Autodesk Inventor part; units mm, degrees
ref_plane "YZ Plane" through (0, 0, 0) normal (1, 0, 0) x (0, 1, 0)
ref_plane "XZ Plane" through (0, 0, 0) normal (0, 1, 0) x (-1, 0, 0)
ref_plane "XY Plane" through (0, 0, 0) normal (0, 0, 1) x (1, 0, 0)
sketch "Sketch1" plane through (0, 0, 0) normal (0, 1, 0) x (-1, 0, 0)
  line L0 (-3, -29) -> (3, -29)
  line L1 (3, -29) -> (3, 29)
  line L2 (3, 29) -> (-3, 29)
  line L3 (-3, 29) -> (-3, -29)
  line L4 (-3, -29) -> (3, 29) construction
  line L5 (3, -29) -> (-3, 29) construction
  point P0 (0, 0)
  dimension "d0" = 58
  dimension "d1" = 6
extrude "Main Body Extrusion" add sketch "Sketch1" along normal blind 4
sketch "Sketch2" plane through (0, 4, 0) normal (0, 1, 0) x (1, 0, 0)
  line L0 (-3, 29) -> (-3, -29)
  line L1 (3, -29) -> (3, 29)
  line L2 (-3, -29) -> (3, -29)
  line L3 (3, -29) -> (3, -23)
  line L4 (3, -23) -> (-3, -23)
  line L5 (-3, -23) -> (-3, -29)
  line L6 (3, 29) -> (-3, 29)
  line L7 (-3, 29) -> (3, 29)
  line L8 (3, 29) -> (3, 23)
  line L9 (3, 23) -> (-3, 23)
  line L10 (-3, 23) -> (-3, 29)
  point P0 (0, 0)
  dimension "d4" = 6
  dimension "d5" = 6
  dimension "d6" = 6
  dimension "d7" = 6
  dimension "d8" = 6
extrude "Side Beams Extrusion" add sketch "Sketch2" along normal blind 20 contours L6 L1 L9 L0 | L4 L1 L2 L0
sketch "Sketch3" plane through (0, 24, 0) normal (0, 1, 0) x (1, 0, 0)
  line L0 (-3, 23) -> (-3, -23)
  line L1 (3, -23) -> (3, 23)
  circle A0 centre (0, 26) radius 2
  line L2 (-3, 23) -> (3, 23)
  line L3 (3, 29) -> (-3, 29)
  circle A1 centre (0, -26) radius 2
  line L4 (-3, -29) -> (3, -29)
  line L5 (3, -29) -> (3, -23)
  point P0 (0, 0)
  dimension "d11" = 6
  dimension "d12" = 4
  dimension "d13" = 3
  dimension "d14" = 6
  dimension "d15" = 3
  dimension "d16" = 4
  dimension "d17" = 3
  dimension "d18" = 3
extrude "Extrusion3" cut sketch "Sketch3" against normal blind 7
fillet "Fillet1" radius 2 10 edges at (-3, 14, -23) (-3, 12, -29) (-3, 4, 0) (3, 4, 0) (-3, 12, 29) (-3, 14, 23) (3, 12, 29) (3, 14, -23) (3, 12, -29) (3, 14, 23)
equation "\"d5\" = d4"
equation "\"d6\" = d4"
equation "\"d7\" = d4"
equation "\"d8\" = d4"
equation "\"d13\" = 0.5 * d14"
equation "\"d15\" = 0.5 * d11"
equation "\"d17\" = d13"
equation "\"d18\" = d15"
properties part number "Battery Holder"
Work out the finished part from the listing and answer in its coordinate system (mm). A direction names the side the tool comes from. Round coordinates to 2 decimals unless told otherwise and drop trailing zeros. Write each loop counter-clockwise with the first axis right and the second up, starting at its lowest first coordinate (ties: lowest second). Pieces come first, ordered by that corner, then holes. Notation, with made-up numbers: M -6.75,1 L 51.25,1 A29 cw 51.25,33 Z; hole C 57,82.25 d7. An arc over 180 degrees is marked long. Use a Markdown table: item, result.
1) A flat-ended cylindrical pin translates along its axis: pin 1 (0.6 mm diameter, centred on x = -0.5, z = -9.5, fed in from +Y). Find the tip coordinate at first contact, or state that the pin passes through.
Taken from the geometry:
| item | result |
|---|---|
| pin 1 | stops at y = 4 |
2) The part is cut by section C-C on x = 0. Give the vertices of the cut face in (y, z), plus the area to 3 significant figures.
Taken from the geometry:
| item | result |
|---|---|
| outline | M 0,-29 L 24,-29 L 24,-28 L 17,-28 L 17,-24 L 24,-24 L 24,-23 L 4,-23 L 4,23 L 24,23 L 24,24 L 17,24 L 17,28 L 24,28 L 24,29 L 0,29 Z |
| area | 416 mm2 |
3) The part is cut by section B-B on y = 9.75. Give the vertices of the cut face in (x, z).
Taken from the geometry:
| item | result |
|---|---|
| outline | M -3,-27 A2 ccw -1,-29 L 1,-29 A2 ccw 3,-27 L 3,-25 A2 ccw 1,-23 L -1,-23 A2 ccw -3,-25 Z; M -3,25 A2 ccw -1,23 L 1,23 A2 ccw 3,25 L 3,27 A2 ccw 1,29 L -1,29 A2 ccw -3,27 Z |
4) The part is cut by section A-A on z = 26. Give the vertices of the cut face in (x, y).
Taken from the geometry:
| item | result |
|---|---|
| outline | M -3,0 L 3,0 L 3,24 L 2,24 L 2,17 L -2,17 L -2,24 L -3,24 Z |
5) Determine the mould class of faces 1 (the face through (2.43, 12.17, -28.4)), 2 (the face through (2.4, 13.15, -23.57)), 3 (the face through (0, 17, 26)), 4 (the face through (2.43, 11.83, 28.4)) for opening direction Z: pulls with the +Z half, pulls with the -Z half, needs draft (parallel to the pull), parting line crosses it, or undercut.
Taken from the geometry:
| item | result |
|---|---|
| face 1 | pulls with the -Z half |
| face 2 | undercut |
| face 3 | undercut |
| face 4 | pulls with the +Z half |
6) The part is cut by section D-D on y = 2.75. Give the vertices of the cut face in (x, z).
Taken from the geometry:
| item | result |
|---|---|
| outline | M -3,-27 A2 ccw -1,-29 L 1,-29 A2 ccw 3,-27 L 3,-25 A2 ccw 2.85,-24.25 L 2.85,24.25 A2 ccw 3,25 L 3,27 A2 ccw 1,29 L -1,29 A2 ccw -3,27 L -3,25 A2 ccw -2.85,24.25 L -2.85,-24.25 A2 ccw -3,-25 Z |
7) Which of the six approach directions +Z, -Z, +X, -X, +Y, -Y give full straight-line access (tool end or side, diameter ignored) to faces 5 (the face through (0, 14, -23)), 6 (the face through (0, 21, -24)), 7 (the face through (-2.43, 13.15, -23.6))?
Taken from the geometry:
| item | result |
|---|---|
| face 5 | +X, -X, +Y |
| face 6 | +Y |
| face 7 | -X, +Y |
8) Consider line 1 (Z direction, x = -0.2, y = 18.5); line 2 (Z direction, x = 0.2, y = 16); line 3 (Y direction, x = 0.25, z = 1.5). Determine where each line is inside the solid, lowest interval first. Write a range as [from, to].
Taken from the geometry:
| item | result |
|---|---|
| line 1 | z = [-29, -27.99], [-24.01, -23], [23, 24.01], [27.99, 29] |
| line 2 | z = [-29, -23], [23, 29] |
| line 3 | y = [0, 4] |
